Work out the finished part from the listing and answer in its coordinate system (mm). Face numbers are marked on the shaded views. Give positions to 0.01 mm unless a question says otherwise; leave off trailing zeros. Loops run counter-clockwise (first coordinate to the right, second up) from the corner with the lowest first, then second, coordinate; pieces in that order, holes last. Notation, with made-up numbers: M 77,-18.75 L 97,-18.75 A21 cw 97,-4.75 Z; hole C -21,43.5 d7. An arc over 180 degrees is marked long. Write item = value, one per line. Start each with the question number.
1. The mould has two halves that part along X. Classify the marked faces 1, 2 and 3: released by +X, released by -X, zero draft, split by the parting line, or undercut.
2. Section A-A on z = 0 is taken. Determine the outline of the cut face in (x, y), plus the area to 4 significant figures.
3. Section D-D on x = 22 is taken. Determine the outline of the cut face in (y, z), plus the area to 3 significant figures.
4. Section B-B on x = 50 is taken. Determine the outline of the cut face in (y, z), plus the area to 3 significant figures.
5. Section C-C on y = 0 is taken. Determine the outline of the cut face in (x, z).
6. Flat-ended cylindrical pins translate along their axes: pin 1 Ø2 at (y, z) = (-1.5, -2.5) entering from -X; pin 2 Ø1.4 at (y, z) = (3, -0.5) entering from +X; pin 3 Ø3 at (x, y) = (20.5, -2.5) entering from +Z; pin 4 Ø3 at (x, y) = (25, 2.5) entering from -Z. Find the tip coordinate at first contact, or state that the pin passes through.
7. Consider L1, parallel to X at y = 0.3, z = 0; L2, parallel to Y at x = 8.5, z = -2.25; L3, parallel to X at y = -1, z = -2. Determine where each line is inside the solid, lowest interval first. Write a range as [from, to].
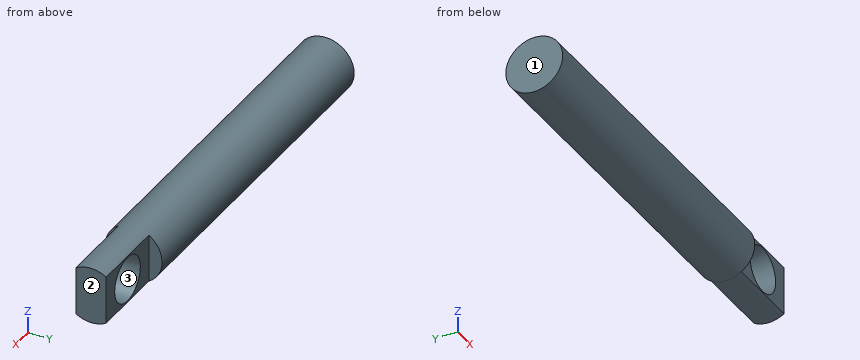
```python
from build123d import *

# Parameters (mm, degrees)
SKETCH1_R           = 3.75
BOSS_EXTRUDE1_DEPTH = 45
BOSS_EXTRUDE2_DEPTH = 10
SKETCH3_R           = 3
CUT_EXTRUDE1_DEPTH  = 10


with BuildPart() as part:
    # Sketch1 → Boss-Extrude1 (new body)
    with BuildSketch(Plane(origin=(0, 0, 0), x_dir=(0, 0, -1), z_dir=(1, 0, 0))):
        with Locations(Location((0, 0, 0), (0, 0, 180))):
            Circle(SKETCH1_R)
    extrude(amount=BOSS_EXTRUDE1_DEPTH)

    # Sketch2 → Boss-Extrude2 (add)
    with BuildSketch(Plane(origin=(45, 0, 0), x_dir=(0, 0, -1), z_dir=(1, 0, 0))):
        with BuildLine():
            Line((3.172144385, 2), (0, 2))
            Line((0, 2), (-3.172144385, 2))
            ThreePointArc((-3.172144385, 2), (-3.75, 0), (-3.172144385, -2))
            Line((-3.172144385, -2), (3.172144385, -2))
            ThreePointArc((3.172144385, -2), (3.602640798, -1.040903107), (3.75, 0))
            ThreePointArc((3.75, 0), (3.602640798, 1.040903107), (3.172144385, 2))
        make_face()
    extrude(amount=BOSS_EXTRUDE2_DEPTH)

    # Sketch3 → Cut-Extrude1 (cut)
    with BuildSketch(Plane(origin=(0, 2, 0), x_dir=(1, 0, 0), z_dir=(0, 1, 0))):
        with Locations(Location((50, 0, 0), (0, 0, 270))):
            Circle(SKETCH3_R)
    extrude(amount=-CUT_EXTRUDE1_DEPTH, mode=Mode.SUBTRACT)


solid = part.part
```
Verdict:
q1.face_1 = released by -X
q1.face_2 = released by +X
q1.face_3 = undercut
q2.outline = M 0,-3.75 L 45,-3.75 L 45,-2 L 47,-2 L 47,2 L 45,2 L 45,3.75 L 0,3.75 Z; M 53,-2 L 55,-2 L 55,2 L 53,2 Z
q2.area = 353.5 mm2
q3.outline = C 0,0 d7.5
q3.area = 44.2 mm2
q4.outline = M -2,-3.17 A3.75 ccw 2,-3.17 L 2,-3 L -2,-3 Z; M -2,3 L 2,3 L 2,3.17 A3.75 ccw -2,3.17 Z
q4.area = 4.51 mm2
q5.outline = M 0,-3.75 L 55,-3.75 L 55,3.75 L 0,3.75 Z; hole C 50,0 d6
q6.pin_1 = 0
q6.pin_2 = 45
q6.pin_3 = 3.61
q6.pin_4 = -3.61
q7.L1 = [0, 47], [53, 55]
q7.L2 = [-3, 3]
q7.L3 = [0, 47.76], [52.24, 55]
